Source: three-view drawing plus pictorial views. Frame: mm from the lowest corner of the part. A direction names the side the tool comes from. Round coordinates to 2 decimals unless told otherwise and drop trailing zeros. Loops run counter-clockwise (first coordinate to the right, second up) from the corner with the lowest first, then second, coordinate; pieces in that order, holes last. Notation, with made-up numbers: M 7.25,36 L 36.25,36 A28 cw 36.25,70 Z; hole C 69.5,54 d6. An arc over 180 degrees is marked long. Answer as a JSON object with one key per item and string values.
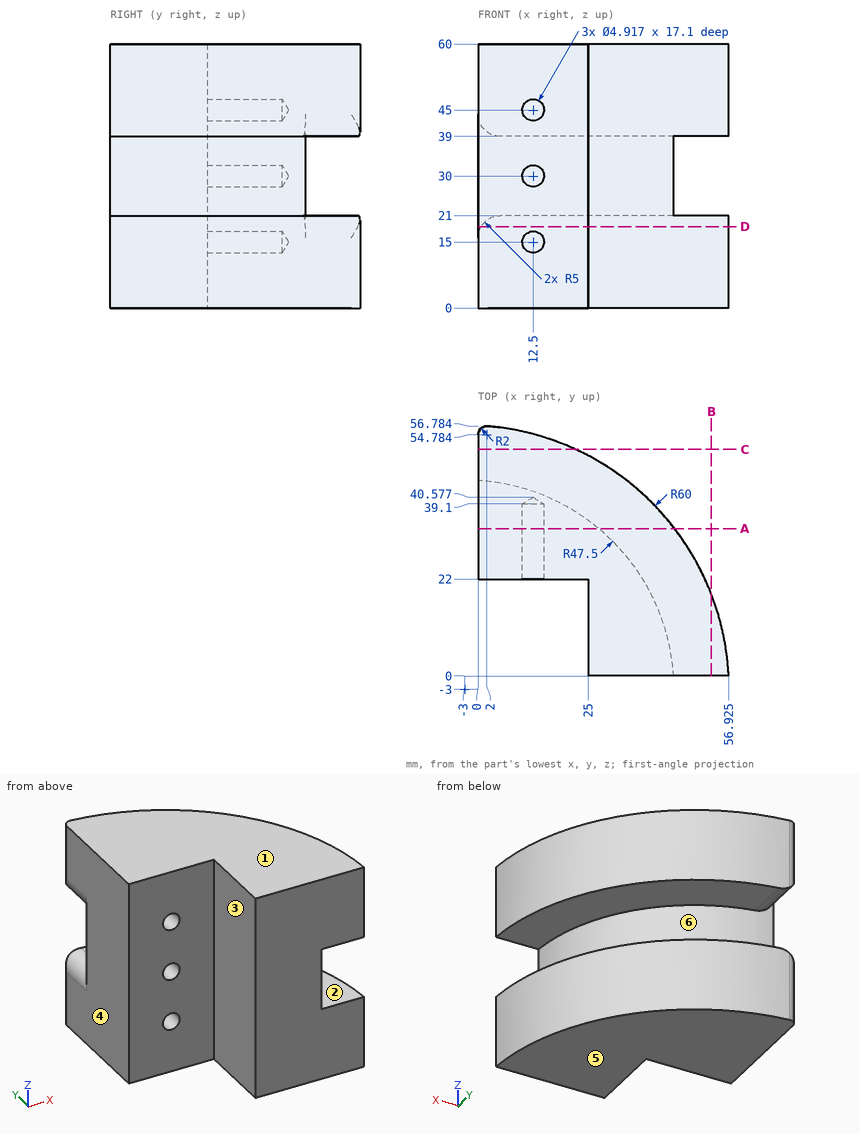
1) Line query: probe 1 along Z at (x, y) = (28.5, 42); probe 2 along Z at (x, y) = (12, 30); probe 3 along X at (y, z) = (35.5, 46.5). Output: solid intervals per line, ascending.
Geometry results:
{"probe 1": "0 to 21, 39 to 60", "probe 2": "0 to 12.59, 17.41 to 27.59, 32.41 to 42.59, 47.41 to 60", "probe 3": "0 to 10.55, 14.45 to 43.02"}
2) First-contact query: pin 1 (12.5 mm diameter, centred on x = 15, z = 39, fed in from -Y); pin 2 (4 mm diameter, centred on x = 12.5, z = 15, fed in from +Y); pin 3 (8 mm diameter, centred on x = 12.5, z = 30, fed in from +Y). Flat tips, straight axial feed; report the tip coordinate or a pass-through.
Geometry results:
{"pin 1": "y = 22", "pin 2": "y = 55.46", "pin 3": "y = 43.09"}
3) Set-up query: the marked faces 1, 2 and 3. Return all of +Z, -Z, +X, -X, +Y, -Y with unobstructed straight access to the full face (end or side cutting, diameter ignored); none if empty.
Geometry results:
{"face 1": "+Z, +X, -X, +Y, -Y", "face 2": "+X, +Y", "face 3": "+Z, -Z, -X, -Y"}
4) Cut plane D-D on z = 18.5. Return the cut outline in (x, y) (1 decimal), and give its area (3 significant figures).
Geometry results:
{"outline": "M 0,22 L 25,22 L 25,0 L 56.9,0 A60 ccw 2.2,56.8 A2 ccw 0.7,56.3 L 0.7,44.4 A47.5 ccw 0,44.4 Z", "area": "1,920 mm2"}
5) Cut plane A-A on y = 33.5. Return the cut outline in (x, z).
Geometry results:
{"outline": "M 0,0 L 44.62,0 L 44.62,21 L 27.4,21 L 27.4,39 L 44.62,39 L 44.62,60 L 0,60 Z; hole C 12.5,15 d4.92; hole C 12.5,30 d4.92; hole C 12.5,45 d4.92"}
6) Cut plane C-C on y = 51.5. Return the cut outline in (x, z) (1 decimal).
Geometry results:
{"outline": "M 0,0 L 22.1,0 L 22.1,21 L 5,21 A5 ccw 0,16 Z; M 0,44 A5 ccw 5,39 L 22.1,39 L 22.1,60 L 0,60 Z"}
7) Pull-direction query (Z, two-part tool) for the marked faces 4, 5 and 6; classes: +Z half, -Z half, draft (parallel to the pull), parting line (faces both ways), or undercut.
Geometry results:
{"face 4": "draft", "face 5": "-Z half", "face 6": "undercut"}
8) Cut plane B-B on x = 53. Return the cut outline in (y, z), and give its area (3 significant figures).
Geometry results:
{"outline": "M 0,0 L 18.54,0 L 18.54,21 L 0,21 Z; M 0,39 L 18.54,39 L 18.54,60 L 0,60 Z", "area": "779 mm2"}
